from build123d import *

# Parameters (mm, degrees)
SKETCH1_W           = 31.86
SKETCH1_H           = 7.81
BOSS_EXTRUDE1_DEPTH = 3.15
SKETCH2_R           = 2.455
BOSS_EXTRUDE2_DEPTH = 1.92
SHELL1_T            = -1.5
SKETCH3_R           = 1.485
SKETCH3_R_2         = 0.565
BOSS_EXTRUDE3_DEPTH = 1.45


with BuildPart() as part:
    # Sketch1 → Boss-Extrude1 (new body)
    with BuildSketch(Plane.XY):
        Rectangle(SKETCH1_W, SKETCH1_H)
    extrude(amount=-BOSS_EXTRUDE1_DEPTH)

    # Sketch2 → Boss-Extrude2 (add)
    with BuildSketch(Plane.XY):
        with Locations((-11.95, 0)):
            Circle(SKETCH2_R)
        with Locations((-3.99, 0)):
            Circle(SKETCH2_R)
        with Locations((3.97, 0)):
            Circle(SKETCH2_R)
        with Locations((11.93, 0)):
            Circle(SKETCH2_R)
    extrude(amount=BOSS_EXTRUDE2_DEPTH)

    # Shell1
    shell1_openings = [part.faces().sort_by_distance(p)[0] for p in [
        (0, 0, -3.15),
    ]]
    offset(amount=SHELL1_T, openings=shell1_openings, kind=Kind.INTERSECTION)

    # Sketch3 → Boss-Extrude3 (add)
    # profile 1 of 3: a face of its own
    with BuildSketch(Plane(origin=(0, 0, -1.5), x_dir=(-1, 0, 0), z_dir=(0, 0, -1))):
        with Locations(Location((-7.965, 0, 0), (0, 0, 180))):
            Circle(SKETCH3_R)
        with Locations(Location((-7.965, 0, 0), (0, 0, 180))):
            Circle(SKETCH3_R_2, mode=Mode.SUBTRACT)
    # profile 2 of 3: a face of its own
    with BuildSketch(Plane(origin=(0, 0, -1.5), x_dir=(-1, 0, 0), z_dir=(0, 0, -1))):
        with Locations(Location((0.005, 0, 0), (0, 0, 180))):
            Circle(SKETCH3_R)
        with Locations(Location((0.005, 0, 0), (0, 0, 180))):
            Circle(SKETCH3_R_2, mode=Mode.SUBTRACT)
    # profile 3 of 3: a face of its own
    with BuildSketch(Plane(origin=(0, 0, -1.5), x_dir=(-1, 0, 0), z_dir=(0, 0, -1))):
        with Locations(Location((7.975, 0, 0), (0, 0, 180))):
            Circle(SKETCH3_R)
        with Locations(Location((7.975, 0, 0), (0, 0, 180))):
            Circle(SKETCH3_R_2, mode=Mode.SUBTRACT)
    extrude(amount=BOSS_EXTRUDE3_DEPTH)


solid = part.part
The listing builds one solid part. Answer for the finished solid, in the listing's coordinates (mm). A direction names the side the tool comes from. Coordinates: 2 decimals unless noted, no trailing zeros. Order: outer loops, then holes, each group sorted by start corner. A loop starts at its lowest first (then second) coordinate and runs counter-clockwise, first axis right, second up.
Q1. A cutting plane is placed at D-D, the plane y = -3.25. Write down the section's boundary in (x, z).
Q2. Which of the six approach directions +Z, -Z, +X, -X, +Y, -Y give full straight-line access (tool end or side, diameter ignored) to faces 1 (the face through (-6.56, -0.45, -2.21)), 2 (the face through (0, 0, 0)), 3 (the face through (12, 0, 1.92))?
Q3. Given P1, Ø0.9, axis at x = 7.965, y = 0, coming from the -Z side; P2, Ø1.5, axis at x = -3.99, y = 0, coming from the -Z side; P3, Ø2.5, axis at x = -8, y = 0.5, coming from the -Z side, each flat-ended and moving along its own axis, determine where each tip first touches the part or whether it passes through.
Q4. A cutting plane is placed at B-B, the plane z = -0.45. Write down the section's boundary in (x, y) (3 decimals).
Q5. A cutting plane is placed at C-C, the plane x = -11.95. Write down the section's boundary in (y, z) (3 decimals), and give its area (3 significant figures).
Q6. Consider line 1 (X direction, y = 0, z = -1.25) (3 decimals); line 2 (X direction, y = 0.75, z = 1.3); line 3 (X direction, y = -2, z = -2.35). Determine where each line is inside the solid, lowest interval first.
Q7. For a pull along Y with two mould halves and no side action, classify faces 4 (the face through (-7, 0, -2.95)), 5 (the face through (0, 3, -3.15)), 6 (the face through (1.517, 0.108, 0.947)) as pulls with the +Y half, pulls with the -Y half, needs draft (parallel to the pull), parting line crosses it, or undercut.
Q8. A cutting plane is placed at A-A, the plane z = -2.05. Write down the section's boundary in (x, y) (3 decimals), and give its area (3 significant figures).
Answers follow:
1. outline: (-15.93, -3.15) - (15.93, -3.15) - (15.93, 0) - (-15.93, 0) - close
2. face 1: -Z
2. face 2: +Z
2. face 3: +Z, +X, -X, +Y, -Y
3. P1: stops at z = -1.5
3. P2: stops at z = 0.42
3. P3: stops at z = -2.95
4. outline: (-15.93, -3.905) - (15.93, -3.905) - (15.93, 3.905) - (-15.93, 3.905) - close; hole circle Ø1.91 at (-11.95, 0); hole circle Ø1.91 at (-3.99, 0); hole circle Ø1.91 at (3.97, 0); hole circle Ø1.91 at (11.93, 0)
5. outline: (-3.905, -3.15) - (-2.405, -3.15) - (-2.405, -1.5) - (-0.955, -1.5) - (-0.955, 0.42) - (0.955, 0.42) - (0.955, -1.5) - (2.405, -1.5) - (2.405, -3.15) - (3.905, -3.15) - (3.905, 0) - (2.455, 0) - (2.455, 1.92) - (-2.455, 1.92) - (-2.455, 0) - (-3.905, 0) - close
5. area: 22.4 mm2
6. line 1: x = -15.93 to -12.905, -10.995 to -4.945, -3.035 to 3.015, 4.925 to 10.975, 12.885 to 15.93
6. line 2: x = -14.29 to -9.61, -6.33 to -1.65, 1.63 to 6.31, 9.59 to 14.27
6. line 3: x = -15.93 to -14.43, 14.43 to 15.93
7. face 4: undercut
7. face 5: needs draft
7. face 6: parting line crosses it
8. outline: (-15.93, -3.905) - (15.93, -3.905) - (15.93, 3.905) - (-15.93, 3.905) - close; circle Ø2.97 at (-7.975, 0); circle Ø2.97 at (-0.005, 0); circle Ø2.97 at (7.965, 0); hole (-14.43, -2.405) - (14.43, -2.405) - (14.43, 2.405) - (-14.43, 2.405) - close; hole circle Ø1.13 at (-7.975, 0); hole circle Ø1.13 at (-0.005, 0); hole circle Ø1.13 at (7.965, 0)
8. area: 128 mm2
